Input: dimensioned drawing with shaded views. Units: mm. Origin: part minimum x, y, z. Give positions to 0.01 mm unless a question says otherwise; leave off trailing zeros. Loops run counter-clockwise (first coordinate to the right, second up) from the corner with the lowest first, then second, coordinate; pieces in that order, holes last.
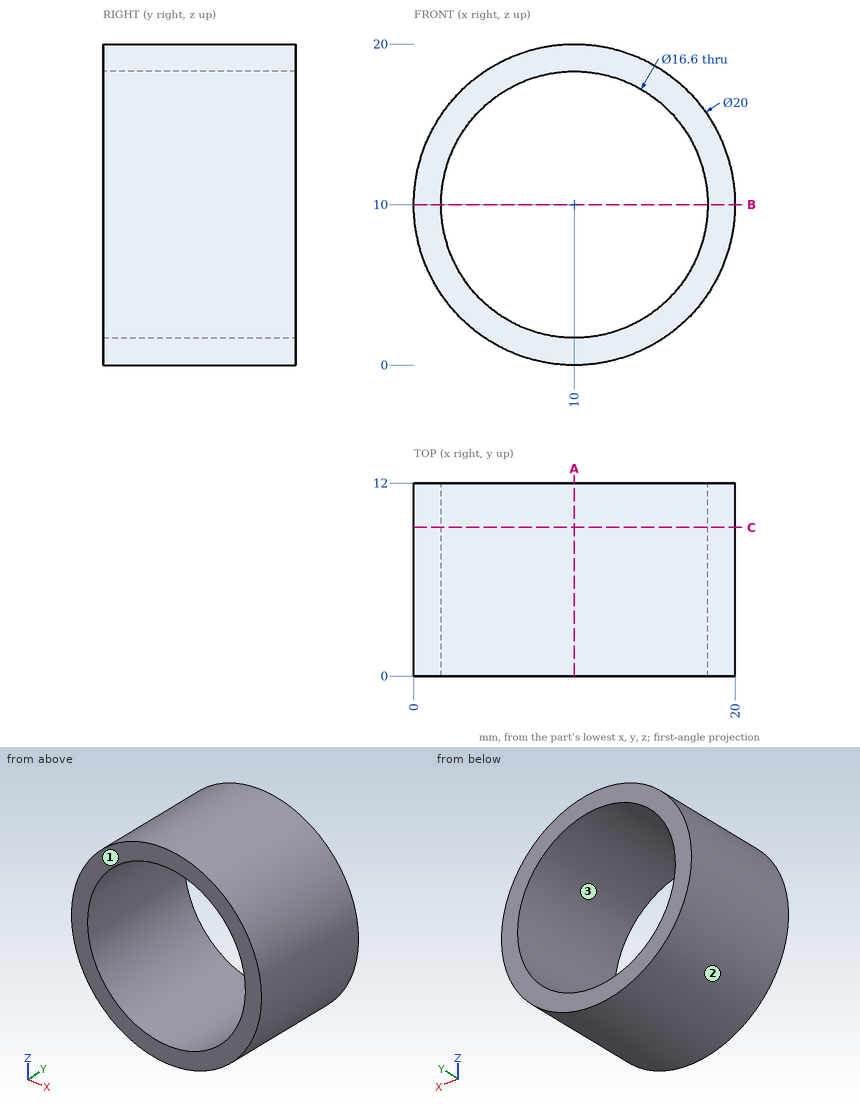
(1) Ray query, line 1 along X through (y, z) = (8.5, 10); line 2 along Z through (x, y) = (2.75, 3.5); line 3 along X through (y, z) = (11, 12). Return the intervals inside material, ascending.
A:
line 1: x = 0 to 1.7, 18.3 to 20
line 2: z = 3.11 to 5.96, 14.04 to 16.89
line 3: x = 0.2 to 1.94, 18.06 to 19.8
(2) Section C-C, the plane y = 9.25. Return the cut outline in (x, z).
A:
outline: circle Ø20 at (10, 10); hole circle Ø16.6 at (10, 10)
(3) Mould query, pull axis X, two halves, no side actions, for the marked faces 1, 2 and 3. Classes: pulls with the +X half, pulls with the -X half, needs draft (parallel to the pull), parting line crosses it, or undercut.
A:
face 1: needs draft
face 2: parting line crosses it
face 3: undercut
(4) Section A-A, the plane x = 10. Return the cut outline in (y, z), then the cut area to 3 significant figures.
A:
outline: (0, 0) - (12, 0) - (12, 1.7) - (0, 1.7) - close; (0, 18.3) - (12, 18.3) - (12, 20) - (0, 20) - close
area: 40.8 mm2
(5) Section B-B, the plane z = 10. Return the cut outline in (x, y), then the cut area to 3 significant figures.
A:
outline: (0, 0) - (1.7, 0) - (1.7, 12) - (0, 12) - close; (18.3, 0) - (20, 0) - (20, 12) - (18.3, 12) - close
area: 40.8 mm2
(6) First-contact query: pin 1 (2 mm diameter, centred on x = 4, y = 10, fed in from +Z); pin 2 (4 mm diameter, centred on x = 17.5, y = 5, fed in from +Z). Flat tips, straight axial feed; report the tip coordinate or a pass-through.
A:
pin 1: stops at z = 18.66
pin 2: stops at z = 18.35
